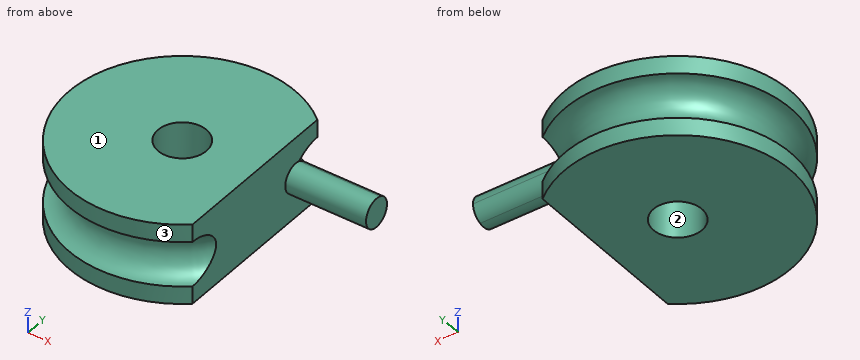
```python
from build123d import *

# Parameters (mm, degrees)
F0_R     = 15
F1_DEPTH = 25
F5_DEPTH = 50


with BuildPart() as f1:
    # F0 (on Top) → F1 (new body, symmetric)
    with BuildSketch(Plane.XY):
        with BuildLine():
            Line((45, -53.6190264738), (45, 53.6190264738))
            ThreePointArc((45, 53.6190264738), (-70, 0), (45, -53.6190264738))
        make_face()
        Circle(F0_R, mode=Mode.SUBTRACT)
    extrude(amount=F1_DEPTH, both=True)

    # F2 (on Right) → F3 (revolve, cut)
    with BuildSketch(Plane.YZ):
        with BuildLine():
            Line((70, -14), (70, 14))
            ThreePointArc((70, 14), (56, 0), (70, -14))
        make_face()
    revolve(axis=Axis((0, 0, 25), (0, 0, 1)), mode=Mode.SUBTRACT)

    # F4 (on face) → F5 (join)
    with BuildSketch(Plane.YZ.offset(45)):
        with BuildLine():
            add(Edge.make_bspline(
                [(37.9630328609, 8.4982607788), (37.8523435019, 8.4048203415), (37.7424820724, 8.3104014762), (37.6334707776, 8.2149986154), (37.525332792, 8.1186060884), (37.4180922716, 8.0212181078), (37.3117743656, 7.9228287563), (37.2064052286, 7.823431974), (36.826236873, 7.4577676485), (36.5572934764, 7.185459665), (36.2956678052, 6.9059722624), (36.041930817, 6.6191996988), (35.7967338532, 6.3250596485), (35.5608040283, 6.0234970289), (35.3349396191, 5.7144878262), (34.9596041272, 5.1618860399), (34.8053000417, 4.9216027682), (34.6574566137, 4.677206923), (34.5164662374, 4.4287401627), (34.3827450871, 4.1762748231), (34.2567257621, 3.9199178725), (34.1388477747, 3.6598159897), (33.972823057, 3.2593369411), (33.9184105228, 3.1215569007), (33.8663694036, 2.9828498623), (33.8167604551, 2.8432475247), (33.769643447, 2.7027852726), (33.7250765475, 2.5615023849), (33.6831157079, 2.4194422423), (33.567344253, 1.998824599), (33.5009341193, 1.7182071188), (33.444986335, 1.43518271), (33.399847873, 1.1501662245), (33.3657973112, 0.8636063961), (33.3430321538, 0.5759874866), (33.331656153, 0.2878309318), (33.3316772398, -0.2920603513), (33.3433625212, -0.5838406442), (33.36672517, -0.8750615205), (33.4016558858, -1.1651818297), (33.4479469745, -1.4536998647), (33.5053059499, -1.7401515835), (33.5733691351, -2.024108832), (33.6915046183, -2.4479228858), (33.7339482932, -2.5899306957), (33.7789927091, -2.7311537294), (33.82658152, -2.8715490352), (33.8766562279, -3.0110777655), (33.9291567963, -3.1497049676), (33.984022265, -3.2873993744), (34.1490037446, -3.6819927579), (34.2650067533, -3.9364311557), (34.3887918355, -4.1872704013), (34.5199466609, -4.4343744462), (34.6580655419, -4.6776436303), (34.8027579562, -4.9170101221), (34.9536551707, -5.1524343498), (35.3248066319, -5.7004684421), (35.5501463092, -6.0096084062), (35.7855690187, -6.3113088937), (36.030274827, -6.6055929723), (36.2835351055, -6.8925150275), (36.5446977166, -7.1721564153), (36.8131911273, -7.4446219389), (37.1944947346, -7.8121861418), (37.3014725192, -7.9132878967), (37.409432192, -8.0133489318), (37.5183462275, -8.1123756019), (37.6281881757, -8.2103741117), (37.7389326494, -8.3073505305), (37.8505553113, -8.403310806), (37.9630328615, -8.4982607786)],
                knots=[0.3142800556, 0.3142800556, 0.3142800556, 0.3142800556, 0.3142800556, 0.3142800556, 0.3142800556, 0.3142800556, 0.3142800556, 0.3358087351, 0.3358087351, 0.3358087351, 0.3358087351, 0.3358087351, 0.3358087351, 0.3358087351, 0.3926809759, 0.3926809759, 0.3926809759, 0.3926809759, 0.3926809759, 0.3926809759, 0.3926809759, 0.43512366, 0.43512366, 0.43512366, 0.43512366, 0.43512366, 0.43512366, 0.43512366, 0.4571495261, 0.4571495261, 0.4571495261, 0.4571495261, 0.4571495261, 0.4571495261, 0.4571495261, 0.5000055628, 0.5000055628, 0.5000055628, 0.5000055628, 0.5000055628, 0.5000055628, 0.5000055628, 0.5434005305, 0.5434005305, 0.5434005305, 0.5434005305, 0.5434005305, 0.5434005305, 0.5434005305, 0.5654393693, 0.5654393693, 0.5654393693, 0.5654393693, 0.5654393693, 0.5654393693, 0.5654393693, 0.6070013278, 0.6070013278, 0.6070013278, 0.6070013278, 0.6070013278, 0.6070013278, 0.6070013278, 0.6638433094, 0.6638433094, 0.6638433094, 0.6638433094, 0.6638433094, 0.6638433094, 0.6638433094, 0.6857197919, 0.6857197919, 0.6857197919, 0.6857197919, 0.6857197919, 0.6857197919, 0.6857197919, 0.6857197919, 0.6857197919], degree=8))
            ThreePointArc((37.9630328609, 8.4982607788), (26, -3e-10), (37.9630328615, -8.4982607786))
        make_face()
        with BuildLine():
            ThreePointArc((37.9630328615, -8.4982607786), (42.3371416694, -5.212135083), (44, 0))
            ThreePointArc((44, 0), (42.3371416692, 5.2121350832), (37.9630328609, 8.4982607788))
            add(Edge.make_bspline(
                [(37.9630328609, 8.4982607788), (37.8523435019, 8.4048203415), (37.7424820724, 8.3104014762), (37.6334707776, 8.2149986154), (37.525332792, 8.1186060884), (37.4180922716, 8.0212181078), (37.3117743656, 7.9228287563), (37.2064052286, 7.823431974), (36.826236873, 7.4577676485), (36.5572934764, 7.185459665), (36.2956678052, 6.9059722624), (36.041930817, 6.6191996988), (35.7967338532, 6.3250596485), (35.5608040283, 6.0234970289), (35.3349396191, 5.7144878262), (34.9596041272, 5.1618860399), (34.8053000417, 4.9216027682), (34.6574566137, 4.677206923), (34.5164662374, 4.4287401627), (34.3827450871, 4.1762748231), (34.2567257621, 3.9199178725), (34.1388477747, 3.6598159897), (33.972823057, 3.2593369411), (33.9184105228, 3.1215569007), (33.8663694036, 2.9828498623), (33.8167604551, 2.8432475247), (33.769643447, 2.7027852726), (33.7250765475, 2.5615023849), (33.6831157079, 2.4194422423), (33.567344253, 1.998824599), (33.5009341193, 1.7182071188), (33.444986335, 1.43518271), (33.399847873, 1.1501662245), (33.3657973112, 0.8636063961), (33.3430321538, 0.5759874866), (33.331656153, 0.2878309318), (33.3316772398, -0.2920603513), (33.3433625212, -0.5838406442), (33.36672517, -0.8750615205), (33.4016558858, -1.1651818297), (33.4479469745, -1.4536998647), (33.5053059499, -1.7401515835), (33.5733691351, -2.024108832), (33.6915046183, -2.4479228858), (33.7339482932, -2.5899306957), (33.7789927091, -2.7311537294), (33.82658152, -2.8715490352), (33.8766562279, -3.0110777655), (33.9291567963, -3.1497049676), (33.984022265, -3.2873993744), (34.1490037446, -3.6819927579), (34.2650067533, -3.9364311557), (34.3887918355, -4.1872704013), (34.5199466609, -4.4343744462), (34.6580655419, -4.6776436303), (34.8027579562, -4.9170101221), (34.9536551707, -5.1524343498), (35.3248066319, -5.7004684421), (35.5501463092, -6.0096084062), (35.7855690187, -6.3113088937), (36.030274827, -6.6055929723), (36.2835351055, -6.8925150275), (36.5446977166, -7.1721564153), (36.8131911273, -7.4446219389), (37.1944947346, -7.8121861418), (37.3014725192, -7.9132878967), (37.409432192, -8.0133489318), (37.5183462275, -8.1123756019), (37.6281881757, -8.2103741117), (37.7389326494, -8.3073505305), (37.8505553113, -8.403310806), (37.9630328615, -8.4982607786)],
                knots=[0.3142800556, 0.3142800556, 0.3142800556, 0.3142800556, 0.3142800556, 0.3142800556, 0.3142800556, 0.3142800556, 0.3142800556, 0.3358087351, 0.3358087351, 0.3358087351, 0.3358087351, 0.3358087351, 0.3358087351, 0.3358087351, 0.3926809759, 0.3926809759, 0.3926809759, 0.3926809759, 0.3926809759, 0.3926809759, 0.3926809759, 0.43512366, 0.43512366, 0.43512366, 0.43512366, 0.43512366, 0.43512366, 0.43512366, 0.4571495261, 0.4571495261, 0.4571495261, 0.4571495261, 0.4571495261, 0.4571495261, 0.4571495261, 0.5000055628, 0.5000055628, 0.5000055628, 0.5000055628, 0.5000055628, 0.5000055628, 0.5000055628, 0.5434005305, 0.5434005305, 0.5434005305, 0.5434005305, 0.5434005305, 0.5434005305, 0.5434005305, 0.5654393693, 0.5654393693, 0.5654393693, 0.5654393693, 0.5654393693, 0.5654393693, 0.5654393693, 0.6070013278, 0.6070013278, 0.6070013278, 0.6070013278, 0.6070013278, 0.6070013278, 0.6070013278, 0.6638433094, 0.6638433094, 0.6638433094, 0.6638433094, 0.6638433094, 0.6638433094, 0.6638433094, 0.6857197919, 0.6857197919, 0.6857197919, 0.6857197919, 0.6857197919, 0.6857197919, 0.6857197919, 0.6857197919, 0.6857197919], degree=8))
        make_face()
    extrude(amount=F5_DEPTH)


solid = f1.part
```
Check sheet for the modelled part. Datum: model origin and axes. Units: mm. Face numbers are marked on the shaded views. Coordinates: 2 decimals unless noted, no trailing zeros. Write each loop counter-clockwise with the first axis right and the second up, starting at its lowest first coordinate (ties: lowest second). Pieces come first, ordered by that corner, then holes. Notation, with made-up numbers: (-6, 56) -> (31, 56) arc R31 ccw to (31, 81) -> close; hole circle Ø8 at (27, 50.5). An arc over 180 degrees is marked (long way). Use a Markdown table: item, result.
1. Sectioned sample at C-C (z = -5). Enter the section's corners in (x, y), plus the area to 3 significant figures.
Reported:
| item | result |
|---|---|
| outline | (45, -34.86) -> (45, 27.52) -> (95, 27.52) -> (95, 42.48) -> (45, 42.48) -> (45, 34.86) arc R56.92 ccw (long way) to start; hole circle Ø30 at (0, 0) |
| area | 9,650 mm2 |
2. Scan lines: line 1 along Y through (x, z) = (8, 2.5); line 2 along Y through (x, z) = (0, 9); line 3 along Z through (x, y) = (29.5, 56.5). Record each from-to range of solid material in increasing order.
Reported:
| item | result |
|---|---|
| line 1 | y = -55.65 to -12.69, 12.69 to 55.65 |
| line 2 | y = -59.28 to -15, 15 to 59.28 |
| line 3 | z = -25 to -12.52, 12.52 to 25 |
3. Sectioned sample at D-D (z = -17.5). Enter the section's corners in (x, y).
Reported:
| item | result |
|---|---|
| outline | (45, -53.62) -> (45, 53.62) arc R70 ccw (long way) to start; hole circle Ø30 at (0, 0) |
4. Sectioned sample at A-A (y = 0). Enter the section's corners in (x, z), plus the area to 3 significant figures.
Reported:
| item | result |
|---|---|
| outline | (-70, -25) -> (-15, -25) -> (-15, 25) -> (-70, 25) -> (-70, 14) arc R14 cw to (-70, -14) -> close; (15, -25) -> (45, -25) -> (45, 25) -> (15, 25) -> close |
| area | 3,940 mm2 |
5. Sectioned sample at B-B (x = 0). Enter the section's corners in (y, z).
Reported:
| item | result |
|---|---|
| outline | (-70, -25) -> (-15, -25) -> (-15, 25) -> (-70, 25) -> (-70, 14) arc R14 cw to (-70, -14) -> close; (15, -25) -> (70, -25) -> (70, -14) arc R14 cw to (70, 14) -> (70, 25) -> (15, 25) -> close |
6. Go/stop test with flat-tipped pins: pin 1 Ø3 at (y, z) = (37.5, -1.5) entering from -X; pin 2 Ø3 at (x, y) = (78.5, 36) entering from +Z; pin 3 Ø1.5 at (y, z) = (-21, -8.5) entering from +X. Record where each tip stops, or that it passes through.
Reported:
| item | result |
|---|---|
| pin 1 | stops at x = -43.02 |
| pin 2 | stops at z = 9 |
| pin 3 | stops at x = 45 |
7. Release check for a two-part mould opening along Y. For the marked faces 1, 2 and 3 record: pulls with the +Y half, pulls with the -Y half, needs draft (parallel to the pull), parting line crosses it, or undercut.
Reported:
| item | result |
|---|---|
| face 1 | needs draft |
| face 2 | undercut |
| face 3 | parting line crosses it |
